```python
from build123d import *

# Parameters (mm, degrees)
F1_DEPTH = 1


# Not quite as in the source:
# - a feature names something its author has since deleted; it is built from what else it names


with BuildPart() as f1:
    # F0 (on Front) → F1 (new body, symmetric)
    with BuildSketch(Plane.XZ):
        with BuildLine():
            ThreePointArc((-58.215127866, 20.8417536759), (-59.5395660257, 10.4582609311), (-59.9821, 0))
            ThreePointArc((-59.9821, 0), (-59.9729371877, -1.5061942231), (-59.9454501071, -3.0121654896))
            ThreePointArc((-59.9454501071, -3.0121654896), (-59.7948238827, -3.3578286914), (-59.4455981282, -3.5))
            Line((-59.4455981282, -3.5), (-56.3175, -3.5))
            ThreePointArc((-56.3175, -3.5), (-55.9639466094, -3.3535533906), (-55.8175, -3))
            Line((-55.8175, -3), (-55.8175, 0.8354))
            ThreePointArc((-55.8175, 0.8354), (-54.9388203436, 2.9567203436), (-52.8175, 3.8354))
            Line((-52.8175, 3.8354), (63.8175, 3.8354))
            ThreePointArc((63.8175, 3.8354), (66.5295373486, 2.7120373486), (67.6529, 0))
            Line((67.6529, 0), (67.6529, -6))
            ThreePointArc((67.6529, -6), (68.9029, -7.25), (70.1529, -6))
            Line((70.1529, -6), (70.1529, 9.2687909752))
            ThreePointArc((70.1529, 9.2687909752), (69.2742203436, 11.3901113188), (67.1529, 12.2687909752))
            Line((67.1529, 12.2687909752), (20.1529, 12.2687909752))
            ThreePointArc((20.1529, 12.2687909752), (18.6529, 13.7687909752), (20.1529, 15.2687909752))
            Line((20.1529, 15.2687909752), (68.1529, 15.2687909752))
            ThreePointArc((68.1529, 15.2687909752), (70.2742203436, 14.3901113188), (71.1529, 12.2687909752))
            Line((71.1529, 12.2687909752), (71.1529, -4.5669872981))
            ThreePointArc((71.1529, -4.5669872981), (71.2779, -4.7834936491), (71.5279, -4.7834936491))
            Line((71.5279, -4.7834936491), (73.0279, -3.9174682453))
            ThreePointArc((73.0279, -3.9174682453), (73.1194063509, -3.8259618943), (73.1529, -3.7009618943))
            Line((73.1529, -3.7009618943), (73.1529, 17.3516533444))
            ThreePointArc((73.1529, 17.3516533444), (72.4019345274, 19.3370610341), (70.5250042038, 20.3284869745))
            Line((70.5250042038, 20.3284869745), (34.3884397258, 24.8455575343))
            ThreePointArc((34.3884397258, 24.8455575343), (33.1504938652, 24.961352042), (31.907745034, 25))
            Line((31.907745034, 25), (-53.2864920761, 25))
            ThreePointArc((-53.2864920761, 25), (-56.510715364, 23.8215682893), (-58.215127866, 20.8417536759))
        make_face()
    extrude(amount=F1_DEPTH, both=True)


solid = f1.part
```
For this review, take the finished solid that the model builds, in its own axes (mm). A direction names the side the tool comes from. Give positions to 0.01 mm unless a question says otherwise; leave off trailing zeros. Loops run counter-clockwise (first coordinate to the right, second up) from the corner with the lowest first, then second, coordinate; pieces in that order, holes last. Notation, with made-up numbers: M 4,14.5 L 37,14.5 A19 ccw 37,29.5 Z; hole C 9.25,-31 d6. An arc over 180 degrees is marked long. One line per item, written item: value. Start each with the question number.
Q1. Machinability: for faces 1 (the face through (52.71, -0.014, 22.555)), 2 (the face through (66.5, -0.01, 2.74)), 3 (the face through (69.297, -0.014, 11.367)), which of the approach directions +Z, -Z, +X, -X, +Y, -Y give a long, thin tool a straight path to every point of the face, cutting with its end or side? Answer none if there is none.
Q2. Add section B-B (z = -1.5). Give the boundary of the cut face in (x, y).
Q3. For L1, parallel to Z at x = -32, y = 0.1; L2, parallel to Z at x = 19, y = 0.7; L3, parallel to Z at x = 39.5, y = -0.9, list the stretches that pass through material, from the lowest coordinate up.
Q4. Clearance check with flat-ended pins moving along their axes: pin 1 Ø0.6 at (x, y) = (33.5, 0) entering from -Z; pin 2 Ø0.6 at (y, z) = (0, 6.5) entering from -X. State where each tip first meets the part, or that it passes through.
Q5. Add section A-A (x = 55.5). Give the boundary of the cut face in (y, z).
Q6. Add section D-D (x = 12). Give the boundary of the cut face in (y, z), and give its area (3 significant figures).
Q7. Draft analysis for pull direction X (two halves, no side actions). For faces 4 (the face through (72.422, -0.014, 19.314)), 5 (the face through (-56.473, -0.014, 23.853)), 6 (the face through (70.251, -0.014, 14.413)), 7 (the face through (6, -1, 13)), state which applies: released by +X, released by -X, zero draft, split by the parting line, or undercut.
Reply:
1. face 1: +Z, +X, +Y, -Y
1. face 2: -Z, +Y, -Y
1. face 3: +Y, -Y
2. outline: M -59.97,-1 L -55.82,-1 L -55.82,1 L -59.97,1 Z; M 67.65,-1 L 70.15,-1 L 70.15,1 L 67.65,1 Z; M 71.15,-1 L 73.15,-1 L 73.15,1 L 71.15,1 Z
3. L1: 3.84 to 25
3. L2: 3.84 to 12.81, 14.73 to 25
3. L3: 3.84 to 12.27, 15.27 to 24.21
4. pin 1: z = 3.84
4. pin 2: x = -59.83
5. outline: M -1,3.84 L 1,3.84 L 1,12.27 L -1,12.27 Z; M -1,15.27 L 1,15.27 L 1,22.21 L -1,22.21 Z
6. outline: M -1,3.84 L 1,3.84 L 1,25 L -1,25 Z
6. area: 42.3 mm²
7. face 4: released by +X
7. face 5: released by -X
7. face 6: undercut
7. face 7: zero draft
